```python
from build123d import *

# Parameters (mm, degrees)
F1_DEPTH  = 12
F3_DEPTH  = 10
F4_R      = 4
F4_R_2    = 5
F5_DEPTH  = 6
F6_R      = 8
F7_R      = 14
F8_R      = 11.235347
F9_DEPTH  = 25
F10_W     = 56.325583
F10_H     = 14
F12_DEPTH = 25
F13_R     = 5


with BuildPart() as f1:
    # F0 (on Top) → F1 (new body)
    with BuildSketch(Plane.XY):
        Polygon((20, 50), (0, 0), (100, 0), (70, 50), (100, 100), (0, 100), align=None)
    extrude(amount=F1_DEPTH)

    # F2 (on face) → F3 (cut)
    with BuildSketch(Plane.XY.offset(12)):
        Polygon((91.169048, 5), (64.169048, 50), (91.169048, 95), (7.385165, 95), (25.385165, 50), (7.385165, 5), align=None)
    extrude(amount=-F3_DEPTH, mode=Mode.SUBTRACT)

    # F4 (on face) → F5 (join)
    with BuildSketch(Plane.XY.offset(2)):
        with Locations((42.898408, 31.41522)):
            Circle(F4_R)
        with Locations((44.494253, 68.297007)):
            Circle(F4_R_2)
    extrude(amount=F5_DEPTH)

    # F6
    f6_edges = [f1.edges().sort_by_distance(p)[0] for p in [
        (7.385165, 95, 7),
        (25.385165, 50, 7),
        (7.385165, 5, 7),
        (91.169048, 95, 7),
        (64.169048, 50, 7),
        (91.169048, 5, 7),
    ]]
    fillet(f6_edges, radius=F6_R)

    # F7
    f7_edges = [f1.edges().sort_by_distance(p)[0] for p in [
        (20, 50, 6),
        (0, 100, 6),
        (100, 100, 6),
        (70, 50, 6),
        (100, 0, 6),
        (0, 0, 6),
    ]]
    fillet(f7_edges, radius=F7_R)

    # F8 (on face) → F9 (cut)
    with BuildSketch(Plane.XY.offset(2)):
        with Locations((43.759387, 50.048411)):
            Circle(F8_R)
    extrude(amount=-F9_DEPTH, mode=Mode.SUBTRACT)

    # F10 (on face) → F12 (cut)
    with BuildSketch(Plane.XY.offset(2)):
        with Locations((45.957904, 16.376337)):
            Rectangle(F10_W, F10_H)
    extrude(amount=-F12_DEPTH, mode=Mode.SUBTRACT)

    # F13
    f13_edges = [f1.edges().sort_by_distance(p)[0] for p in [
        (17.795112, 23.376337, 1),
        (74.120695, 23.376337, 1),
        (74.120695, 9.376337, 1),
        (17.795112, 9.376337, 1),
    ]]
    fillet(f13_edges, radius=F13_R)


solid = f1.part
```
The model under review builds one solid part; all positions refer to its coordinate system, in mm. A direction names the side the tool comes from. Give positions to 0.01 mm unless a question says otherwise; leave off trailing zeros. Write each loop counter-clockwise with the first axis right and the second up, starting at its lowest first coordinate (ties: lowest second). Pieces come first, ordered by that corner, then holes. Notation, with made-up numbers: (-32, -9) - (-24, -9) arc R21 ccw to (-24, 28) - close; hole circle Ø3 at (69, -20.75). An arc over 180 degrees is marked (long way). Answer in a Markdown table with one row per item. Add a question column.
1. Tool access review of faces 1 (the cylindrical face through (87.35, 93.08, 6.08)), 2 (the flat face through (12.73, 68.18, 5.92)), 3 (the cylindrical face through (19.3, 21.95, 0.99)), 4 (the cylindrical face through (12.64, 91.58, 6.93)): name each direction out of +Z, -Z, +X, -X, +Y, -Y from which nothing blocks a thin tool from reaching the whole face with its end or side.
2. Wall thickness on line 1 along Y through (x, z) = (44, 1.25); line 2 along Y through (x, z) = (26.5, 2.25); line 3 along Y through (x, z) = (41, 4.25): over which ranges is each line inside the solid? List them lowest first. Write a range as [from, to].
3. We need section A-A on x = 58. Write out the cut boundary in (y, z).
4. We need section D-D on x = 36. Write out the cut boundary in (y, z).
5. We need section B-B on z = 4.25. Write out the cut boundary in (x, y), then the cut area to 3 significant figures.
6. Insertion check: P1, Ø3, axis at x = 38, y = 72, coming from the -Z side; P2, Ø3, axis at x = 46, y = 70.5, coming from the +Z side; P3, Ø1.6, axis at y = 17.5, z = 1, coming from the +X side; P4, Ø13.5, axis at x = 43.76, y = 50.05, coming from the -Z side. Each pin has a flat end and moves straight along its axis. Give the tip position at first contact, or say it passes through.
7. Draft analysis for pull direction Y (two halves, no side actions). For faces 5 (the cylindrical face through (40.81, 71.68, 4.96)), 6 (the flat face through (47, 62, 0)), 7 (the flat face through (48, 0, 6)), state which applies: +Y half, -Y half, draft (parallel to the pull), parting line (faces both ways), or undercut.
8. We need section C-C on z = 9.5. Write out the cut boundary in (x, y).
Ans:
| question | item | result |
|---|---|---|
| 1 | face 1 | +Z, -Z, +X |
| 1 | face 2 | +Z, -Z, -X |
| 1 | face 3 | +Z, -Z |
| 1 | face 4 | +Z |
| 2 | line 1 | y = [0, 9.38], [23.38, 38.82], [61.28, 100] |
| 2 | line 2 | y = [0, 5], [95, 100] |
| 2 | line 3 | y = [0, 5], [27.89, 34.94], [64.72, 71.87], [95, 100] |
| 3 | outline | (0, 0) - (9.38, 0) - (9.38, 2) - (5, 2) - (5, 12) - (0, 12) - close; (23.38, 0) - (100, 0) - (100, 12) - (95, 12) - (95, 2) - (23.38, 2) - close |
| 4 | outline | (0, 0) - (9.38, 0) - (9.38, 2) - (5, 2) - (5, 12) - (0, 12) - close; (23.38, 0) - (41.92, 0) - (41.92, 2) - (23.38, 2) - close; (58.17, 0) - (100, 0) - (100, 12) - (95, 12) - (95, 2) - (58.17, 2) - close |
| 5 | outline | (7.68, 19.2) arc R14 ccw to (20.68, 0) - (75.27, 0) arc R14 ccw to (87.28, 21.2) - (74.32, 42.8) arc R14 cw to (74.32, 57.2) - (87.28, 78.8) arc R14 ccw to (75.27, 100) - (20.68, 100) arc R14 ccw to (7.68, 80.8) - (17.92, 55.2) arc R14 cw to (17.92, 44.8) - close; circle Ø8 at (42.9, 31.42); circle Ø10 at (44.49, 68.3); hole (11.77, 15.97) arc R8 ccw to (19.2, 5) - (77.04, 5) arc R8 ccw to (83.9, 17.12) - (66.64, 45.88) arc R8 cw to (66.64, 54.12) - (83.9, 82.88) arc R8 ccw to (77.04, 95) - (19.2, 95) arc R8 ccw to (11.77, 84.03) - (24.2, 52.97) arc R8 cw to (24.2, 47.03) - close |
| 5 | area | 1,800 mm^2 |
| 6 | P1 | stops at z = 0 |
| 6 | P2 | stops at z = 8 |
| 6 | P3 | stops at x = 89.01 |
| 6 | P4 | passes through |
| 7 | face 5 | undercut |
| 7 | face 6 | draft |
| 7 | face 7 | -Y half |
| 8 | outline | (7.68, 19.2) arc R14 ccw to (20.68, 0) - (75.27, 0) arc R14 ccw to (87.28, 21.2) - (74.32, 42.8) arc R14 cw to (74.32, 57.2) - (87.28, 78.8) arc R14 ccw to (75.27, 100) - (20.68, 100) arc R14 ccw to (7.68, 80.8) - (17.92, 55.2) arc R14 cw to (17.92, 44.8) - close; hole (11.77, 15.97) arc R8 ccw to (19.2, 5) - (77.04, 5) arc R8 ccw to (83.9, 17.12) - (66.64, 45.88) arc R8 cw to (66.64, 54.12) - (83.9, 82.88) arc R8 ccw to (77.04, 95) - (19.2, 95) arc R8 ccw to (11.77, 84.03) - (24.2, 52.97) arc R8 cw to (24.2, 47.03) - close |
